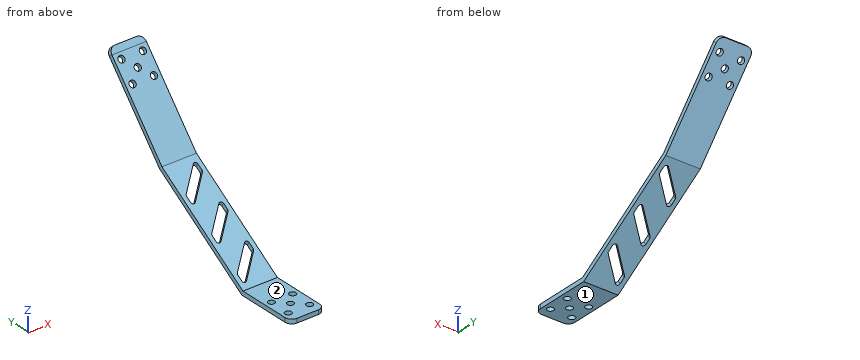
```python
from build123d import *

# Parameters (mm, degrees)
SKETCH_1_W          = 16
SKETCH_1_H          = 48
EXTRUDE_1_DEPTH     = 3
SKETCH_2_R          = 1.5
CUT_EXTRUDE_1_DEPTH = 26.475478406
SKETCH_3_W          = 16
SKETCH_3_H          = 88
EXTRUDE_2_DEPTH     = 3
SKETCH_4_W          = 16
SKETCH_4_H          = 3
EXTRUDE_3_DEPTH     = 2
SKETCH_5_R          = 1.5
CUT_EXTRUDE_2_DEPTH = 108.805767963
FILLET_3_R          = 3
EXTRUDE_4_DEPTH     = 16
CUT_EXTRUDE_3_DEPTH = 111.135894355
CUT_EXTRUDE_4_DEPTH = 111.135894355
CUT_EXTRUDE_5_DEPTH = 110.131666201
FILLET_4_R          = 1


with BuildPart() as part:
    # Sketch 1 → Extrude 1 (new body)
    with BuildSketch(Plane.XY):
        Rectangle(SKETCH_1_W, SKETCH_1_H)
    extrude(amount=EXTRUDE_1_DEPTH)

    # Sketch 2 → Cut-Extrude 1 (cut, through all)
    with BuildSketch(Plane.XY.offset(3)):
        with Locations((-4.949747468, -9.050252532)):
            Circle(SKETCH_2_R)
        with Locations((0, -14)):
            Circle(SKETCH_2_R)
        with Locations((4.949747468, -9.050252532)):
            Circle(SKETCH_2_R)
        with Locations((4.949747468, -18.949747468)):
            Circle(SKETCH_2_R)
        with Locations((-4.949747468, -18.949747468)):
            Circle(SKETCH_2_R)
    extrude(amount=-CUT_EXTRUDE_1_DEPTH, mode=Mode.SUBTRACT)



with BuildPart() as body_2:
    # Sketch 3 → Extrude 2 (new body)
    with BuildSketch(Plane(origin=(0, 12.184675108, -10.591976476), x_dir=(-1, 0, 0), z_dir=(0, 0.7547095802227686, -0.6560590289905112))):
        with Locations((0, 62.009545436)):
            Rectangle(SKETCH_3_W, SKETCH_3_H)
    extrude(amount=EXTRUDE_2_DEPTH)


with BuildPart() as part_1:
    add(part.part)

    add(body_2.part)  # Extrude 3 merges body 2
    # Sketch 4 → Extrude 3 (add)
    with BuildSketch(Plane(origin=(0, 11.815324892, 13.591976476), x_dir=(-1, 0, 0), z_dir=(0, -0.6560590289905113, -0.7547095802227686))):
        with Locations((0, 17.644852838)):
            Rectangle(SKETCH_4_W, SKETCH_4_H)
    extrude(amount=EXTRUDE_3_DEPTH)

    # Sketch 5 → Cut-Extrude 2 (cut, through all)
    with BuildSketch(Plane(origin=(0, 12.184675108, -10.591976476), x_dir=(1, 0, 0), z_dir=(0, -0.7547095802227686, 0.6560590289905113))):
        with Locations(Location((0, 95.34, 0), (0, 0, 270))):
            Circle(SKETCH_5_R)
        with Locations(Location((-4.949747468, 100.289747468, 0), (0, 0, 270))):
            Circle(SKETCH_5_R)
        with Locations(Location((4.949747468, 100.289747468, 0), (0, 0, 270))):
            Circle(SKETCH_5_R)
        with Locations(Location((4.949747468, 90.390252532, 0), (0, 0, 270))):
            Circle(SKETCH_5_R)
        with Locations(Location((-4.949747468, 90.390252532, 0), (0, 0, 270))):
            Circle(SKETCH_5_R)
    extrude(amount=-CUT_EXTRUDE_2_DEPTH, mode=Mode.SUBTRACT)

    # Fillet 3
    fillet_3_edges = [part_1.edges().sort_by_distance(p)[0] for p in [
        (8, 82.865258921, 68.430354516),
        (-8, 82.865258921, 68.430354516),
        (8, -24, 1.5),
        (-8, -24, 1.5),
    ]]
    fillet(fillet_3_edges, radius=FILLET_3_R)

    # Sketch 6 → Extrude 4 (add)
    with BuildSketch(Plane.ZY.offset(8)):
        Polygon((33.531489951, 50.5406193), (3, 3.472509188), (0, 4.360298556), (31.244508057, 52.52761525), align=None)
    extrude(amount=-EXTRUDE_4_DEPTH)

    # Sketch 9 → Cut-Extrude 3 (cut, through all)
    with BuildSketch(Plane(origin=(8, 0, 0), x_dir=(0, 0, -1), z_dir=(1, 0, 0))):
        Polygon((0, 4.360298556), (-31.244508057, 52.52761525), (6.052752185, 30.680291416), align=None)
    extrude(amount=-CUT_EXTRUDE_3_DEPTH, mode=Mode.SUBTRACT)

    # Sketch 11 → Cut-Extrude 4 (cut, through all)
    with BuildSketch(Plane.ZY.offset(8)):
        Polygon((33.531489951, 50.5406193), (3, 3.472509188), (3, -21), (2, -21), (2, -26.591575896), (76.346344159, 89.084017238), (66.49425529, 80.519727044), (67.150314319, 79.765017464), align=None)
        Polygon((66.49425529, 80.519727044), (32.769162653, 51.202951283), (33.531489951, 50.5406193), (67.150314319, 79.765017464), align=None)
        Polygon((32.769162653, 51.202951283), (2, 3.768438978), (3, 3.472509188), (33.531489951, 50.5406193), align=None)
        Polygon((3, 3.472509188), (2, 3.768438978), (2, -21), (3, -21), align=None)
    extrude(amount=-CUT_EXTRUDE_4_DEPTH, mode=Mode.SUBTRACT)

    # Sketch 12 → Cut-Extrude 5 (cut, through all)
    with BuildSketch(Plane(origin=(0, 1.291325132, -1.990739187), x_dir=(-1, 0, 0), z_dir=(0, 0.5442014418825505, -0.8389545819965185))):
        Polygon((-6, 53.414735581), (6, 41.414735581), (6, 47.07158983), (-6, 59.07158983), align=None)
        Polygon((-6, 17.658092453), (6, 5.658092453), (6, 11.314946702), (-6, 23.314946702), align=None)
        Polygon((-6, 35.536414017), (6, 23.536414017), (6, 29.193268266), (-6, 41.193268266), align=None)
    extrude(amount=-CUT_EXTRUDE_5_DEPTH, mode=Mode.SUBTRACT)

    # Fillet 4
    fillet_4_edges = [part_1.edges().sort_by_distance(p)[0] for p in [
        (6, 50.305504644, 30.995059755),
        (-6, 40.23804966, 24.464642452),
        (-6, 35.492205868, 21.386174213),
        (6, 45.559660852, 27.916591516),
        (6, 35.306404849, 21.265651381),
        (-6, 20.493106073, 11.656765839),
        (-6, 25.238949865, 14.735234079),
        (6, 30.560561057, 18.187183142),
        (6, 20.307305055, 11.536243007),
        (-6, 10.239850071, 5.005825705),
        (-6, 5.494006278, 1.927357466),
        (6, 15.561461262, 8.457774768),
    ]]
    fillet(fillet_4_edges, radius=FILLET_4_R)


solid = part_1.part
```
Geometry: final body of the model. Coordinates: model frame, mm. Face numbers are marked on the shaded views. A direction names the side the tool comes from. Coordinates: 2 decimals unless noted, no trailing zeros. Order: outer loops, then holes, each group sorted by start corner. A loop starts at its lowest first (then second) coordinate and runs counter-clockwise, first axis right, second up. Notation, with made-up numbers: M -1,-16 L 13,-16 A9 cw 13,-11 Z; hole C 37.25,50.25 d3. An arc over 180 degrees is marked long. Answer in a Markdown table with one row per item. Add a question column.
Q1. Section query A-A on y = -14. Return the cut outline in (x, z).
Q2. Section query B-B on x = 0. Return the cut outline in (y, z), and give its area (3 significant figures).
Q3. Reachability of the marked faces 1 and 2 from +Z, -Z, +X, -X, +Y, -Y: full face, straight path, thin tool, end or side. Return the list, or none.
Q4. Line query: L1, parallel to X at y = 74, z = 56.5; L2, parallel to Z at x = -2.75, y = -15; L3, parallel to X at y = 48.5, z = 29. Output: solid intervals per line, ascending.
Q5. Contact query for flat-ended pins moving along their axis: P1, Ø4, axis at x = -3.5, z = 13, coming from the -Y side; P2, Ø4, axis at x = -4.95, y = -18.95, coming from the +Z side; P3, Ø8, axis at x = 1.5, z = 51.5, coming from the -Y side. Output: stop coordinate, or through.
Q6. Section query D-D on y = 58.5. Return the cut outline in (x, z), and give its area (3 significant figures).
Q7. Section query C-C on z = 36. Return the cut outline in (x, y).
Completed:
| question | item | result |
|---|---|---|
| 1 | outline | M -8,0 L -1.5,0 L -1.5,2 L -8,2 Z; M 1.5,0 L 8,0 L 8,2 L 1.5,2 Z |
| 2 | outline | M -24,0 L -15.5,0 L -15.5,2 L -24,2 Z; M -12.5,0 L 4.36,0 L 11.07,4.35 L 9.98,6.03 L 3.77,2 L -12.5,2 Z; M 14.73,9.11 L 15.82,7.43 L 26.07,14.08 L 24.98,15.76 Z; M 29.73,18.84 L 30.82,17.16 L 41.07,23.81 L 39.98,25.49 Z; M 44.73,28.57 L 45.82,26.89 L 52.53,31.24 L 76.01,58.26 L 74.5,59.57 L 51.2,32.77 Z; M 76.47,61.84 L 77.98,60.53 L 84,67.45 L 82.49,68.76 Z |
| 2 | area | 220 mm2 |
| 3 | face 1 | -Z, +X, -X, +Y, -Y |
| 3 | face 2 | +Z, +X, -X, -Y |
| 4 | L1 | x = -8 to -6.22, -3.68 to 3.68, 6.22 to 8 |
| 4 | L2 | z = 0 to 2 |
| 4 | L3 | x = -8 to 3.4, 6 to 8 |
| 5 | P1 | stops at y = 17.64 |
| 5 | P2 | stops at z = 2 |
| 5 | P3 | stops at y = 64.01 |
| 6 | outline | M -8,38.11 L 8,38.11 L 8,41.16 L -8,41.16 Z |
| 6 | area | 48.8 mm2 |
| 7 | outline | M -8,54.01 L 8,54.01 L 8,56.66 L -8,56.66 Z |
